Build history of the part. All positions in model axes, mm. Face numbers are marked on the shaded views. A direction names the side the tool comes from. Give positions to 0.01 mm unless a question says otherwise; leave off trailing zeros. Order: outer loops, then holes, each group sorted by start corner. A loop starts at its lowest first (then second) coordinate and runs counter-clockwise, first axis right, second up. Notation, with made-up numbers: (-9, 87.25) - (19, 87.25) arc R23 ccw to (19, 123.25) - close; hole circle Ø7 at (71.25, -37.5). An arc over 180 degrees is marked (long way). Use a Markdown table: item, result. Add a question column.
(1) Mould opens along Y. For the marked faces 1, 2 and 3 say: +Y half, -Y half, draft (parallel to the pull), parting line (faces both ways), or undercut.
(2) Wall check: line 1 (Z direction, x = -9.5, y = 5.25); line 2 (Y direction, x = -1.55, z = 11); line 3 (Y direction, x = -1.85, z = 6.5). Give the ranges that are in metal, low to high.
(3) Slice it at C-C (x = -26). Write the cut outline in (y, z).
(4) Flat gauge pins, fed straight in: pin 1 (2.5 mm diameter, centred on y = 0, z = 11, fed in from -X); pin 2 (5.5 mm diameter, centred on y = 0, z = 6.5, fed in from +X). Where does each tip first touch, or does it go through?
(5) Slice it at D-D (y = -5). Write the cut outline in (x, z).
(6) Slice it at A-A (y = 0). Write the cut outline in (x, z).
(7) Which spindle directions (+Z, -Z, +X, -X, +Y, -Y) get a long thin tool onto all of the face, cutting with end or side? Do the marked faces 4 and 5. Say none if no direction does.
(8) Slice it at B-B (z = 11). Write the cut outline in (x, y), then the cut area to 3 significant figures.
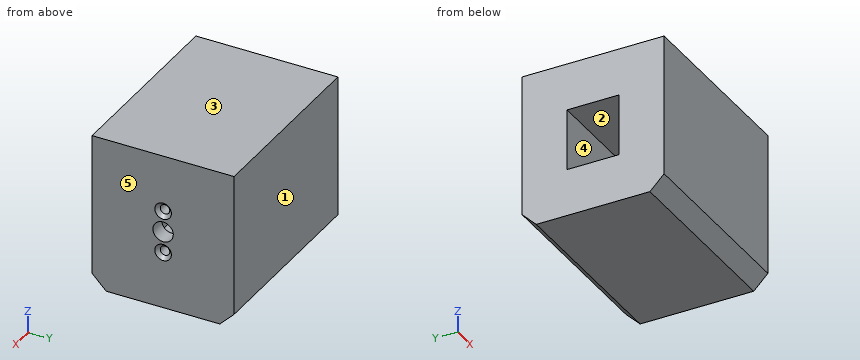
from build123d import *

# Parameters (mm, degrees)
BOSS_EXTRUDE1_DEPTH                             = 23
BOSS_EXTRUDE1_DEPTH_BACK                        = 10
SKETCH1_W                                       = 36.6
SKETCH1_H                                       = 11
SKETCH1_5_W                                     = 36.6
SKETCH1_5_H                                     = 11
CUT_EXTRUDE1_DEPTH                              = 13
SKETCH2_R                                       = 2.15
CUT_EXTRUDE2_DEPTH                              = 46.755436835
CSK_FOR_M2_FLAT_HEAD_MACHINE_SCREW1_D           = 2
CSK_FOR_M2_FLAT_HEAD_MACHINE_SCREW1_CSINK_D     = 3.5
CSK_FOR_M2_FLAT_HEAD_MACHINE_SCREW1_CSINK_ANGLE = 90
CHAMFER1_SIZE                                   = 3


with BuildPart() as part:
    # Sketch1 → Boss-Extrude1 (new, two sides: drawn at the far end of the back side and taken through both)
    with BuildSketch(Plane.XY.offset(-BOSS_EXTRUDE1_DEPTH_BACK)):
        Polygon((0, 15), (-40, 15), (-40, 5.5), (-3.4, 5.5), (-3.4, -5.5), (-40, -5.5), (-40, -15), (0, -15), align=None)
        with Locations((-21.7, 0)):
            Rectangle(SKETCH1_W, SKETCH1_H)
    extrude(amount=BOSS_EXTRUDE1_DEPTH + BOSS_EXTRUDE1_DEPTH_BACK)

    # Sketch1_5 → Cut-Extrude1 (cut)
    with BuildSketch(Plane.XY):
        with Locations((-21.7, 0)):
            Rectangle(SKETCH1_5_W, SKETCH1_5_H)
    extrude(amount=CUT_EXTRUDE1_DEPTH, mode=Mode.SUBTRACT)

    # Sketch2 → Cut-Extrude2 (cut, through all)
    with BuildSketch(Plane.ZY.offset(3.4)):
        with Locations((6.5, 0)):
            Circle(SKETCH2_R)
    extrude(amount=-CUT_EXTRUDE2_DEPTH, mode=Mode.SUBTRACT)

    # CSK for M2 Flat Head Machine Screw1 (through all)
    with Locations(Plane(origin=(0, 0, 0), x_dir=(0, 0, -1), z_dir=(1, 0, 0))):
        with Locations((-11, 0), (-2, 0)):
            CounterSinkHole(CSK_FOR_M2_FLAT_HEAD_MACHINE_SCREW1_D / 2, CSK_FOR_M2_FLAT_HEAD_MACHINE_SCREW1_CSINK_D / 2, counter_sink_angle=CSK_FOR_M2_FLAT_HEAD_MACHINE_SCREW1_CSINK_ANGLE)

    # Chamfer1
    chamfer1_edges = [part.edges().sort_by_distance(p)[0] for p in [
        (-20, -15, -10),
        (-20, 15, -10),
    ]]
    chamfer(chamfer1_edges, length=CHAMFER1_SIZE)


solid = part.part
Solution:
| question | item | result |
|---|---|---|
| 1 | face 1 | +Y half |
| 1 | face 2 | undercut |
| 1 | face 3 | draft |
| 2 | line 1 | -10 to 0, 13 to 23 |
| 2 | line 2 | -15 to -1, 1 to 15 |
| 2 | line 3 | -15 to -2.15, 2.15 to 15 |
| 3 | outline | (-15, -7) - (-12, -10) - (12, -10) - (15, -7) - (15, 23) - (-15, 23) - close; hole (-5.5, 0) - (5.5, 0) - (5.5, 13) - (-5.5, 13) - close |
| 4 | pin 1 | x = -3.4 |
| 4 | pin 2 | x = 0 |
| 5 | outline | (-40, -10) - (0, -10) - (0, 23) - (-40, 23) - (-40, 13) - (-3.4, 13) - (-3.4, 0) - (-40, 0) - close |
| 6 | outline | (-40, -10) - (0, -10) - (0, 0.25) - (-0.75, 1) - (-3.4, 1) - (-3.4, 0) - (-40, 0) - close; (-40, 13) - (-3.4, 13) - (-3.4, 12) - (-0.75, 12) - (0, 12.75) - (0, 23) - (-40, 23) - close; (-3.4, 3) - (-0.75, 3) - (0, 3.75) - (0, 4.35) - (-3.4, 4.35) - close; (-3.4, 8.65) - (0, 8.65) - (0, 9.25) - (-0.75, 10) - (-3.4, 10) - close |
| 7 | face 4 | -X |
| 7 | face 5 | +Z, -Z, +X, +Y, -Y |
| 8 | outline | (-40, -15) - (0, -15) - (0, -1.75) - (-0.75, -1) - (-3.4, -1) - (-3.4, -5.5) - (-40, -5.5) - close; (-40, 5.5) - (-3.4, 5.5) - (-3.4, 1) - (-0.75, 1) - (0, 1.75) - (0, 15) - (-40, 15) - close |
| 8 | area | 790 mm2 |
